The figure shows three views and two pictorial views of one solid part (mm, origin at its lowest corner). Answer the questions. A direction names the side the tool comes from. Coordinates: 2 decimals unless noted, no trailing zeros. Loops run counter-clockwise (first coordinate to the right, second up) from the corner with the lowest first, then second, coordinate; pieces in that order, holes last. Notation, with made-up numbers: (-2, 6) - (37, 6) arc R36 cw to (37, 45) - close; hole circle Ø5 at (-30.5, 33.5). An arc over 180 degrees is marked (long way). One line per question, with ' | ' between items.
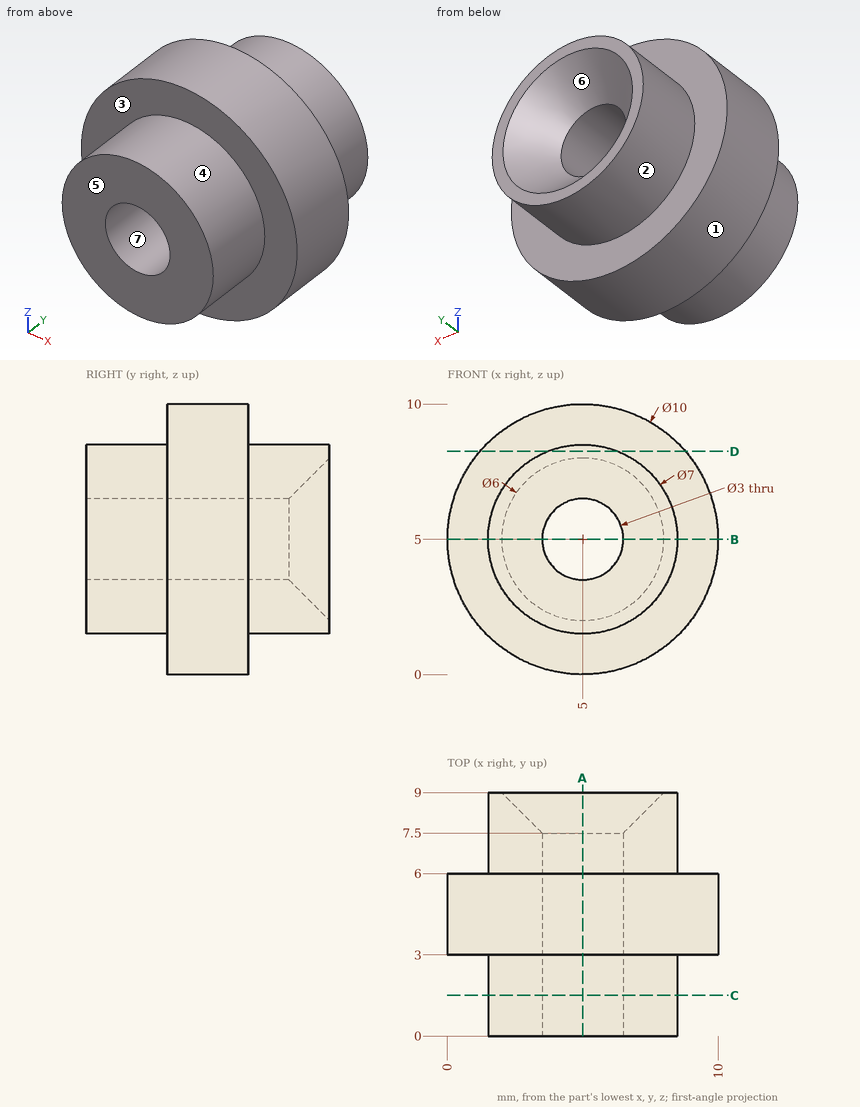
Item 1: Each of these flat-tipped pins is pushed along its axis until it touches: pin 1 Ø1 at (x, y) = (7.5, 1.5) entering from +Z; pin 2 Ø2.5 at (x, z) = (5, 5) entering from -Y. Where does it stop, or does it pass through?
Taken from the geometry:
pin 1: stops at z = 7.87 | pin 2: passes through
Item 2: Find section D-D, the plane z = 8.25. Write down the section's boundary in (x, y).
Taken from the geometry:
outline: (1.2, 3) - (3.7, 3) - (3.7, 0) - (6.3, 0) - (6.3, 3) - (8.8, 3) - (8.8, 6) - (6.3, 6) - (6.3, 9) - (3.7, 9) - (3.7, 6) - (1.2, 6) - close
Item 3: The mould has two halves that part along Z. Classify the marked faces 4, 5, 6 and 7: pulls with the +Z half, pulls with the -Z half, needs draft (parallel to the pull), parting line crosses it, or undercut.
Taken from the geometry:
face 4: parting line crosses it | face 5: needs draft | face 6: undercut | face 7: undercut
Item 4: Find section C-C, the plane y = 1.5. Write down the section's boundary in (x, z), plus the area to 3 significant figures.
Taken from the geometry:
outline: circle Ø7 at (5, 5); hole circle Ø3 at (5, 5) | area: 31.4 mm2
Item 5: Find section B-B, the plane z = 5. Write down the section's boundary in (x, y).
Taken from the geometry:
outline: (0, 3) - (1.5, 3) - (1.5, 0) - (3.5, 0) - (3.5, 7.5) - (2, 9) - (1.5, 9) - (1.5, 6) - (0, 6) - close; (6.5, 0) - (8.5, 0) - (8.5, 3) - (10, 3) - (10, 6) - (8.5, 6) - (8.5, 9) - (8, 9) - (6.5, 7.5) - close
Item 6: Which of the six approach directions +Z, -Z, +X, -X, +Y, -Y give full straight-line access (tool end or side, diameter ignored) to the marked faces 1, 2 and 3?
Taken from the geometry:
face 1: +Y, -Y | face 2: +Y | face 3: -Y
Item 7: Find section A-A, the plane x = 5. Write down the section's boundary in (y, z), plus the area to 4 significant figures.
Taken from the geometry:
outline: (0, 1.5) - (3, 1.5) - (3, 0) - (6, 0) - (6, 1.5) - (9, 1.5) - (9, 2) - (7.5, 3.5) - (0, 3.5) - close; (0, 6.5) - (7.5, 6.5) - (9, 8) - (9, 8.5) - (6, 8.5) - (6, 10) - (3, 10) - (3, 8.5) - (0, 8.5) - close | area: 42.75 mm2
Item 8: Find the intervals of material crossed by line 1 (X direction, y = 2, z = 5); line 2 (Z direction, x = 5, y = 5), in increasing order. Write a range as [from, to].
Taken from the geometry:
line 1: x = [1.5, 3.5], [6.5, 8.5] | line 2: z = [0, 3.5], [6.5, 10]
